from build123d import *

# Parameters (mm, degrees)
SKETCH1_R           = 110.567781149
BOSS_EXTRUDE1_DEPTH = 25.4
SKETCH2_R           = 19.05
SKETCH2_R_2         = 9.525
CUT_EXTRUDE3_DEPTH  = 140.716
CUT_EXTRUDE4_DEPTH  = 134.112
SKETCH6_W           = 10.16
SKETCH6_H           = 7.62


with BuildPart() as part:
    # Sketch1 → Boss-Extrude1 (new body)
    with BuildSketch(Plane.XY):
        Circle(SKETCH1_R)
    extrude(amount=BOSS_EXTRUDE1_DEPTH)

    # Sketch2 → Cut-Extrude3 (cut)
    with BuildSketch(Plane.XY.offset(25.4)):
        with Locations((0, 63.5)):
            Circle(SKETCH2_R)
        with Locations((63.5, 0)):
            Circle(SKETCH2_R)
        with Locations((44.901280605, -44.901280605)):
            Circle(SKETCH2_R_2)
        with Locations((0, -63.5)):
            Circle(SKETCH2_R)
        with Locations((44.901280605, 44.901280605)):
            Circle(SKETCH2_R_2)
        with Locations((-44.901280605, -44.901280605)):
            Circle(SKETCH2_R_2)
        with Locations((-63.5, 0)):
            Circle(SKETCH2_R)
        with Locations((-44.901280605, 44.901280605)):
            Circle(SKETCH2_R_2)
    extrude(amount=-CUT_EXTRUDE3_DEPTH, mode=Mode.SUBTRACT)

    # Sketch5 → Cut-Extrude4 (cut)
    with BuildSketch(Plane.XY.offset(25.4)):
        with BuildLine():
            Line((-3.175, 10.16), (3.175, 10.16))
            Line((3.175, 10.16), (3.175, 5.588))
            ThreePointArc((3.175, 5.588), (0, -6.427003112), (-3.175, 5.588))
            Line((-3.175, 5.588), (-3.175, 10.16))
        make_face()
    extrude(amount=-CUT_EXTRUDE4_DEPTH, mode=Mode.SUBTRACT)

    # Sketch6 → Cut-Revolve1 (revolve, cut)
    with BuildSketch(Plane(origin=(0, 0, 0), x_dir=(0, 0, -1), z_dir=(1, 0, 0))):
        with Locations((-12.7, 106.757781149)):
            Rectangle(SKETCH6_W, SKETCH6_H)
    revolve(axis=Axis((0, 0, 0), (0, 0, 1)), mode=Mode.SUBTRACT)


solid = part.part
For this review, take the finished solid that the model builds, in its own axes (mm). A direction names the side the tool comes from. Round coordinates to 2 decimals unless told otherwise and drop trailing zeros. Loops run counter-clockwise (first coordinate to the right, second up) from the corner with the lowest first, then second, coordinate; pieces in that order, holes last. Notation, with made-up numbers: (-29, -37) - (-17, -37) arc R22 ccw to (-17, -5) - close; hole circle Ø3 at (6.5, 15.25). An arc over 180 degrees is marked (long way). One line per item, written item: value. Start each with the question number.
Item 1: The part is to be moulded in two halves that separate along X. For faces 3 (the flat face through (0, 10.16, 13)), 4 (the flat face through (23, 2, 0)), 5 (the cylindrical face through (-30.9, 98.2, 12.6)), say which applies: +X half, -X half, draft (parallel to the pull), parting line (faces both ways), or undercut.
Item 2: Clearance check with flat-ended pins moving along their axes: pin 1 Ø4 at (x, z) = (-18, 11) entering from +Y; pin 2 Ø5 at (x, z) = (-1.5, 13.5) entering from -Y; pin 3 Ø3 at (y, z) = (83, 15) entering from -X; pin 4 Ø25 at (x, y) = (-44.9, 44.9) entering from +Z. State where each tip first meets the part, or that it passes through.
Item 3: For L1, parallel to Y at x = 0, z = 19.25; L2, parallel to X at y = 7, z = 22.75 (3 decimals); L3, parallel to Y at x = 8, z = 18, list the stretches that pass through material, from the lowest coordinate up.
Item 4: Take a section at B-B (y = 0). Give the boundary of the cut face in (x, z).
Item 5: Take a section at D-D (x = -63.5). Give the boundary of the cut face in (y, z).
Item 6: Take a section at A-A (x = 0). Give the boundary of the cut face in (y, z), plus the area to 3 significant figures.
Item 7: Take a section at C-C (z = 12.75). State how many separate pieces and enclosed holes the cut face has, plus the area to 3 significant figures.
Item 8: For faces 1 (the flat face through (-50, 91, 17.78)), 2 (the cylindrical face through (0.236, -6.423, 12.878)), list the 3-axis set-ups (+Z, -Z, +X, -X, +Y, -Y) from which the entire face can be reached by the end or side of a thin tool; tool diameter is ignored.
Answer below:
1. face 3: undercut
1. face 4: draft
1. face 5: parting line
2. pin 1: stops at y = 101.7
2. pin 2: stops at y = -102.95
2. pin 3: stops at x = -62.9
2. pin 4: stops at z = 25.4
3. L1: y = -110.57 to -82.55, -44.45 to -6.43, 10.16 to 44.45, 82.55 to 110.57
3. L2: x = -110.346 to -81.217, -45.783 to -3.175, 3.175 to 45.783, 81.217 to 110.346
3. L3: y = -110.28 to -80.79, -46.21 to 46.21, 80.79 to 110.28
4. outline: (-110.57, 0) - (-82.55, 0) - (-82.55, 25.4) - (-110.57, 25.4) - (-110.57, 17.78) - (-102.95, 17.78) - (-102.95, 7.62) - (-110.57, 7.62) - close; (-44.45, 0) - (-6.43, 0) - (-6.43, 25.4) - (-44.45, 25.4) - close; (6.43, 0) - (44.45, 0) - (44.45, 25.4) - (6.43, 25.4) - close; (82.55, 0) - (110.57, 0) - (110.57, 7.62) - (102.95, 7.62) - (102.95, 17.78) - (110.57, 17.78) - (110.57, 25.4) - (82.55, 25.4) - close
5. outline: (-90.52, 0) - (-19.05, 0) - (-19.05, 25.4) - (-90.52, 25.4) - (-90.52, 17.78) - (-81.03, 17.78) - (-81.03, 7.62) - (-90.52, 7.62) - close; (19.05, 0) - (90.52, 0) - (90.52, 7.62) - (81.03, 7.62) - (81.03, 17.78) - (90.52, 17.78) - (90.52, 25.4) - (19.05, 25.4) - close
6. outline: (-110.57, 0) - (-82.55, 0) - (-82.55, 25.4) - (-110.57, 25.4) - (-110.57, 17.78) - (-102.95, 17.78) - (-102.95, 7.62) - (-110.57, 7.62) - close; (-44.45, 0) - (-6.43, 0) - (-6.43, 25.4) - (-44.45, 25.4) - close; (10.16, 0) - (44.45, 0) - (44.45, 25.4) - (10.16, 25.4) - close; (82.55, 0) - (110.57, 0) - (110.57, 7.62) - (102.95, 7.62) - (102.95, 17.78) - (110.57, 17.78) - (110.57, 25.4) - (82.55, 25.4) - close
6. area: 3,110 mm2
7. separate pieces: 1
7. enclosed holes: 9
7. area: 27,400 mm2
8. face 1: none
8. face 2: +Z, -Z
